Check sheet for the drawn part. Datum: minimum x, y, z corner. Units: mm. A direction names the side the tool comes from. Round coordinates to 2 decimals unless told otherwise and drop trailing zeros. Write each loop counter-clockwise with the first axis right and the second up, starting at its lowest first coordinate (ties: lowest second). Pieces come first, ordered by that corner, then holes. Notation, with made-up numbers: (-37.5, -33) - (14.5, -33) arc R26 ccw to (14.5, -2) - close; hole circle Ø6 at (0, -31.5). An arc over 180 degrees is marked (long way). Answer as a JSON object with one key per item and string values.
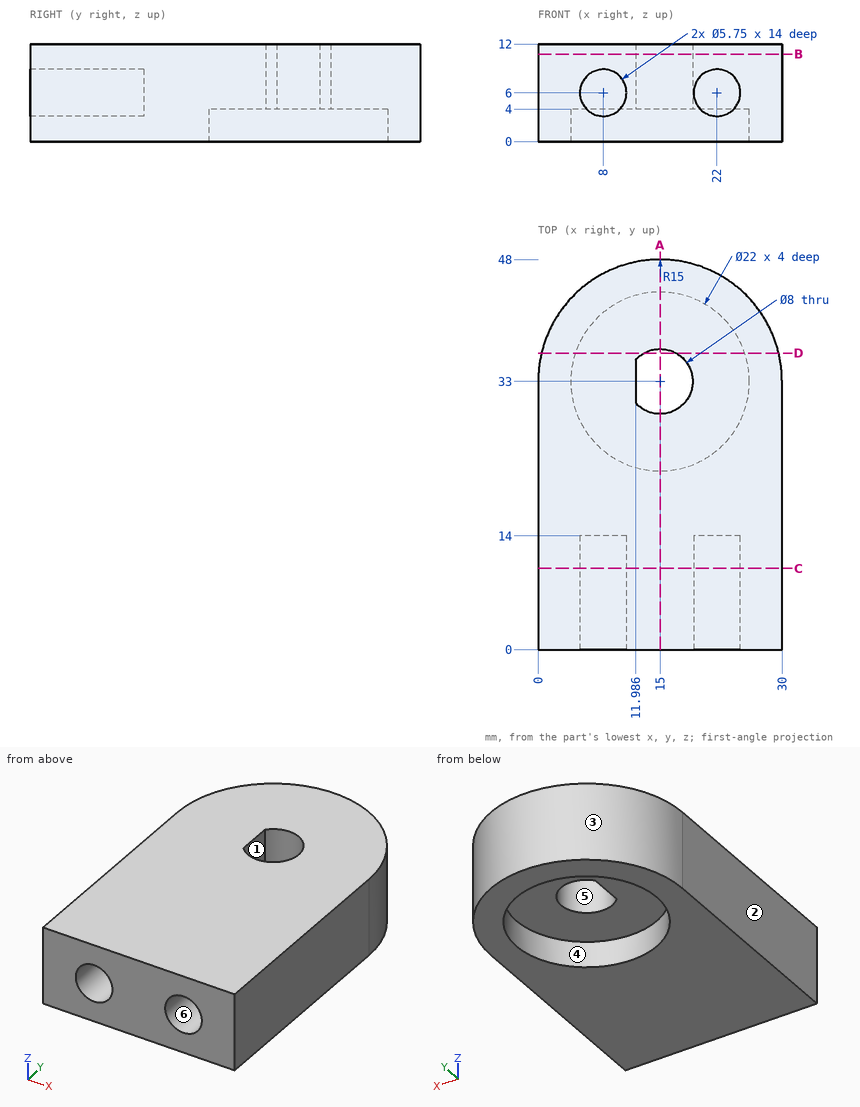
1. Cross-section at B-B (z = 10.75). Record the boundary of the cut face in (x, y).
Completed:
{"outline": "(0, 0) - (30, 0) - (30, 33) arc R15 ccw to (0, 33) - close; hole (11.99, 30.37) arc R4 ccw (long way) to (11.99, 35.63) - close"}
2. Material ranges on probe 1 along Z at (x, y) = (22, 3.75) (3 decimals); probe 2 along X at (y, z) = (9, 4.5); probe 3 along X at (y, z) = (9.5, 3.75), recorded low to high. Write a range as from..to.
Completed:
{"probe 1": "z = 0..3.125, 8.875..12", "probe 2": "x = 0..5.55, 10.45..19.55, 24.45..30", "probe 3": "x = 0..6.21, 9.79..20.21, 23.79..30"}
3. Go/stop test with flat-tipped pins: pin 1 (17.5 mm diameter, centred on x = 15, y = 33, fed in from -Z); pin 2 (4.5 mm diameter, centred on x = 8, z = 5.5, fed in from -Y). Record where each tip stops, or that it passes through.
Completed:
{"pin 1": "stops at z = 4", "pin 2": "stops at y = 14"}
4. Cross-section at D-D (y = 36.5). Record the boundary of the cut face in (x, z), plus the area to 3 significant figures.
Completed:
{"outline": "(0.41, 0) - (4.57, 0) - (4.57, 4) - (13.06, 4) - (13.06, 12) - (0.41, 12) - close; (16.94, 4) - (25.43, 4) - (25.43, 0) - (29.59, 0) - (29.59, 12) - (16.94, 12) - close", "area": "236 mm^2"}
5. Access from +Z, -Z, +X, -X, +Y, -Y to the whole of each face (thin tool, end or side, straight path). Record for the marked faces 4, 5 and 6.
Completed:
{"face 4": "-Z", "face 5": "+Z, -Z", "face 6": "-Y"}
6. Cross-section at C-C (y = 10). Record the boundary of the cut face in (x, z) (3 decimals), plus the area to 3 significant figures.
Completed:
{"outline": "(0, 0) - (30, 0) - (30, 12) - (0, 12) - close; hole circle Ø5.75 at (8, 6); hole circle Ø5.75 at (22, 6)", "area": "308 mm^2"}
7. Mould release check, pull along Y, two halves, no side actions. Record for the marked faces 1, 2 and 3: released by +Y, released by -Y, zero draft, split by the parting line, or undercut.
Completed:
{"face 1": "undercut", "face 2": "zero draft", "face 3": "released by +Y"}
8. Cross-section at A-A (x = 15). Record the boundary of the cut face in (y, z).
Completed:
{"outline": "(0, 0) - (22, 0) - (22, 4) - (29, 4) - (29, 12) - (0, 12) - close; (37, 4) - (44, 4) - (44, 0) - (48, 0) - (48, 12) - (37, 12) - close"}
